```python
from build123d import *

# Parameters (mm, degrees)
BOSS_EXTRUDE1_OUTLINE_R = 1.75
BOSS_EXTRUDE1_DEPTH     = 4
CUT_EXTRUDE1_DEPTH      = 1


# Read off the part's stored shape, not the designer's step: Boss-Extrude1
with BuildPart() as part:
    # Boss-Extrude1 outline → Boss-Extrude1 (new body)
    with BuildSketch(Plane(origin=(0, 0, 0), x_dir=(1, 0, 0), z_dir=(0, 1, 0))):
        with BuildLine():
            Line((25.516474615, -10.33744254), (37.54307775, -10.33744254))
            ThreePointArc((37.54307775, -10.33744254), (39.979776182, -5.587442326), (42.416474615, -10.33744254))
            Line((42.416474615, -10.33744254), (49.479776182, -10.33744254))
            Line((49.479776182, -10.33744254), (49.479776182, -18.81631662))
            Line((49.479776182, -18.81631662), (58.854776182, -18.81631662))
            Line((58.854776182, -18.81631662), (58.854776182, -4.977921711))
            Line((58.854776182, -4.977921711), (-21.145223818, -4.977921711))
            Line((-21.145223818, -4.977921711), (-21.145223818, -18.81631662))
            Line((-21.145223818, -18.81631662), (-11.770223818, -18.81631662))
            Line((-11.770223818, -18.81631662), (-11.770223818, -10.33744254))
            Line((-11.770223818, -10.33744254), (3.74307775, -10.33744254))
            ThreePointArc((3.74307775, -10.33744254), (6.179776182, -5.587442326), (8.616474615, -10.33744254))
            Line((8.616474615, -10.33744254), (20.64307775, -10.33744254))
            ThreePointArc((20.64307775, -10.33744254), (23.079776182, -5.587442326), (25.516474615, -10.33744254))
        make_face()
        with Locations((-16.145223818, -13.587442433)):
            Circle(BOSS_EXTRUDE1_OUTLINE_R, mode=Mode.SUBTRACT)
        with Locations((53.854776182, -13.587442433)):
            Circle(BOSS_EXTRUDE1_OUTLINE_R, mode=Mode.SUBTRACT)
    extrude(amount=BOSS_EXTRUDE1_DEPTH)

    # Sketch2 → Cut-Extrude1 (cut)
    with BuildSketch(Plane(origin=(0, 4, 0), x_dir=(1, 0, 0), z_dir=(0, 1, 0))):
        Polygon((-18.749121586, -7.085274104), (-17.202326714, -7.085274104), (-17.202326714, -7.655145899), (-18.179249791, -7.655145899), (-18.179249791, -8.265722822), (-17.202326714, -8.265722822), (-17.202326714, -8.835594617), (-18.179249791, -8.835594617), (-18.179249791, -10.260274104), (-18.749121586, -10.260274104), align=None)
        Polygon((-16.826440296, -7.085274104), (-16.15480568, -7.085274104), (-15.491439294, -8.104810362), (-14.826800873, -7.085274104), (-14.153258204, -7.085274104), (-15.154985969, -8.621256676), (-14.088384406, -10.260274104), (-14.760019022, -10.260274104), (-15.491439294, -9.136430955), (-16.224131602, -10.260274104), (-16.897038253, -10.260274104), (-15.827256602, -8.619984641), align=None)
    extrude(amount=-CUT_EXTRUDE1_DEPTH, mode=Mode.SUBTRACT)


solid = part.part
```
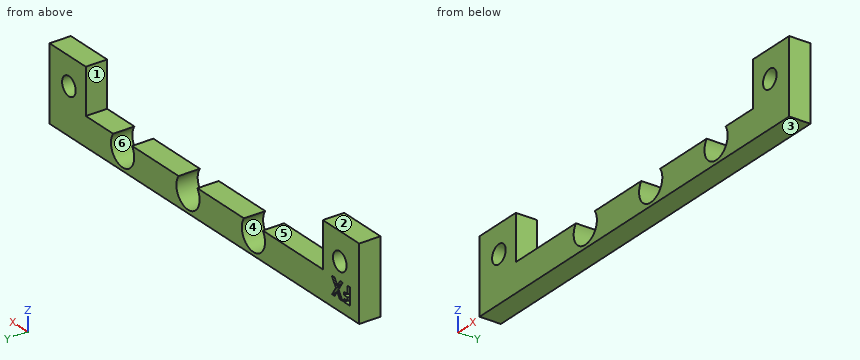
The listing builds one solid part. Answer for the finished solid, in the listing's coordinates (mm). Face numbers are marked on the shaded views. A direction names the side the tool comes from. Round coordinates to 2 decimals unless told otherwise and drop trailing zeros. Loops run counter-clockwise (first coordinate to the right, second up) from the corner with the lowest first, then second, coordinate; pieces in that order, holes last.
1) Consider line 1 (X direction, y = 2.35, z = 13.75); line 2 (X direction, y = 0.35, z = 14.5); line 3 (X direction, y = 1.1, z = 15.75). Determine where each line is inside the solid, lowest interval first.
Outcome:
line 1: x = -21.15 to -17.89, -14.4 to -11.77, 49.48 to 52.11, 55.6 to 58.85
line 2: x = -21.15 to -17.64, -14.65 to -11.77, 49.48 to 52.36, 55.35 to 58.85
line 3: x = -21.15 to -11.77, 49.48 to 58.85
2) For a pull along Z with two mould halves and no side action, classify the marked faces 1, 2, 3 and 4 as released by +Z, released by -Z, zero draft, split by the parting line, or undercut.
Outcome:
face 1: zero draft
face 2: released by +Z
face 3: released by -Z
face 4: undercut
3) Given P1, Ø2, axis at x = 29.5, y = 2.5, coming from the +Z side; P2, Ø3, axis at x = -16.15, z = 13.59, coming from the +Y side, each flat-ended and moving along its own axis, determine where each tip first touches the part or whether it passes through.
Outcome:
P1: stops at z = 10.34
P2: passes through
4) A cutting plane is placed at D-D on y = 1.35. Determine the outline of the cut face in (x, z).
Outcome:
outline: (-21.15, 4.98) - (58.85, 4.98) - (58.85, 18.82) - (49.48, 18.82) - (49.48, 10.34) - (42.42, 10.34) arc R3 cw (long way) to (37.54, 10.34) - (25.52, 10.34) arc R3 cw (long way) to (20.64, 10.34) - (8.62, 10.34) arc R3 cw (long way) to (3.74, 10.34) - (-11.77, 10.34) - (-11.77, 18.82) - (-21.15, 18.82) - close; hole circle Ø3.5 at (-16.15, 13.59); hole circle Ø3.5 at (53.85, 13.59)
5) A cutting plane is placed at B-B on z = 12.5. Determine the outline of the cut face in (x, y), plus the area to 3 significant figures.
Outcome:
outline: (-21.15, 0) - (-17.52, 0) - (-17.52, 4) - (-21.15, 4) - close; (-14.77, 0) - (-11.77, 0) - (-11.77, 4) - (-14.77, 4) - close; (49.48, 0) - (52.48, 0) - (52.48, 4) - (49.48, 4) - close; (55.23, 0) - (58.85, 0) - (58.85, 4) - (55.23, 4) - close
area: 53.1 mm2
6) A cutting plane is placed at C-C on x = 53. Determine the outline of the cut face in (y, z), plus the area to 3 significant figures.
Outcome:
outline: (0, 4.98) - (4, 4.98) - (4, 12.06) - (0, 12.06) - close; (0, 15.11) - (4, 15.11) - (4, 18.82) - (0, 18.82) - close
area: 43.1 mm2
7) A cutting plane is placed at A-A on z = 16.5. Determine the outline of the cut face in (x, y).
Outcome:
outline: (-21.15, 0) - (-11.77, 0) - (-11.77, 4) - (-21.15, 4) - close; (49.48, 0) - (58.85, 0) - (58.85, 4) - (49.48, 4) - close
8) For the marked faces 5 and 6, determine the directions among +Z, -Z, +X, -X, +Y, -Y from which every point of the face is accessible in a straight line to the end or side of a thin tool.
Outcome:
face 5: +Z, +Y, -Y
face 6: +Y, -Y
